Design review of the part built by this model. Coordinates are the model's own, in mm. A direction names the side the tool comes from. Coordinates: 2 decimals unless noted, no trailing zeros. Order: outer loops, then holes, each group sorted by start corner. A loop starts at its lowest first (then second) coordinate and runs counter-clockwise, first axis right, second up. Notation, with made-up numbers: (-27, 0) -> (29, 0) arc R36 cw to (29, 35) -> close; hole circle Ø1 at (69.5, -33). An arc over 180 degrees is marked (long way). Write item = value, one per line.
```python
from build123d import *

# Parameters (mm, degrees)
SKETCH1_R           = 27.5
BOSS_EXTRUDE1_DEPTH = 3
SKETCH2_R           = 27.5
SKETCH2_R_2         = 24.5
BOSS_EXTRUDE2_DEPTH = 15
SKETCH4_R           = 4
CUT_EXTRUDE1_DEPTH  = 5
SKETCH5_R           = 1.5
CUT_EXTRUDE2_DEPTH  = 10
FILLET1_R           = 2
SKETCH6_R           = 24.5
SKETCH6_R_2         = 22.5
BOSS_EXTRUDE3_DEPTH = 20


with BuildPart() as part:
    # Sketch1 → Boss-Extrude1 (new body)
    with BuildSketch(Plane(origin=(0, 0, 0), x_dir=(1, 0, 0), z_dir=(0, 1, 0))):
        with Locations(Location((0, 0, 0), (0, 0, 270))):
            Circle(SKETCH1_R)
    extrude(amount=BOSS_EXTRUDE1_DEPTH)

    # Sketch2 → Boss-Extrude2 (add)
    with BuildSketch(Plane(origin=(0, 3, 0), x_dir=(1, 0, 0), z_dir=(0, 1, 0))):
        with Locations(Location((0, 0, 0), (0, 0, 270))):
            Circle(SKETCH2_R)
        with Locations(Location((0, 0, 0), (0, 0, 270))):
            Circle(SKETCH2_R_2, mode=Mode.SUBTRACT)
    extrude(amount=BOSS_EXTRUDE2_DEPTH)

    # Sketch4 → Cut-Extrude1 (cut)
    with BuildSketch(Plane(origin=(0, 3, 0), x_dir=(1, 0, 0), z_dir=(0, 1, 0))):
        with Locations(Location((0, 0, 0), (0, 0, 270))):
            Circle(SKETCH4_R)
    extrude(amount=-CUT_EXTRUDE1_DEPTH, mode=Mode.SUBTRACT)

    # Sketch5 → Cut-Extrude2 (cut)
    with BuildSketch(Plane(origin=(0, 3, 0), x_dir=(1, 0, 0), z_dir=(0, 1, 0))):
        with BuildLine():
            Line((-2.588190451, 9.659258263), (-5.176380902, 19.318516526))
            ThreePointArc((-5.176380902, 19.318516526), (-14.142135624, 14.142135624), (-19.318516526, 5.176380902))
            Line((-19.318516526, 5.176380902), (-9.659258263, 2.588190451))
            ThreePointArc((-9.659258263, 2.588190451), (-7.071067812, 7.071067812), (-2.588190451, 9.659258263))
        make_face()
        with BuildLine():
            ThreePointArc((19.318516526, 5.176380902), (14.142135624, 14.142135624), (5.176380902, 19.318516526))
            Line((5.176380902, 19.318516526), (2.588190451, 9.659258263))
            ThreePointArc((2.588190451, 9.659258263), (7.071067812, 7.071067812), (9.659258263, 2.588190451))
            Line((9.659258263, 2.588190451), (19.318516526, 5.176380902))
        make_face()
        with BuildLine():
            Line((-9.659258263, -2.588190451), (-19.318516526, -5.176380902))
            ThreePointArc((-19.318516526, -5.176380902), (-14.142135624, -14.142135624), (-5.176380902, -19.318516526))
            Line((-5.176380902, -19.318516526), (-2.588190451, -9.659258263))
            ThreePointArc((-2.588190451, -9.659258263), (-7.071067812, -7.071067812), (-9.659258263, -2.588190451))
        make_face()
        with BuildLine():
            ThreePointArc((5.176380902, -19.318516526), (14.142135624, -14.142135624), (19.318516526, -5.176380902))
            Line((19.318516526, -5.176380902), (9.659258263, -2.588190451))
            ThreePointArc((9.659258263, -2.588190451), (7.071067812, -7.071067812), (2.588190451, -9.659258263))
            Line((2.588190451, -9.659258263), (5.176380902, -19.318516526))
        make_face()
        with Locations(Location((0, 15, 0), (0, 0, 270))):
            Circle(SKETCH5_R)
        with Locations(Location((15, 0, 0), (0, 0, 270))):
            Circle(SKETCH5_R)
        with Locations(Location((0, -15, 0), (0, 0, 270))):
            Circle(SKETCH5_R)
        with Locations(Location((-15, 0, 0), (0, 0, 270))):
            Circle(SKETCH5_R)
    extrude(amount=-CUT_EXTRUDE2_DEPTH, mode=Mode.SUBTRACT)

    # Fillet1
    fillet1_edges = [part.edges().sort_by_distance(p)[0] for p in [
        (-9.659258263, 1.5, 2.588190451),
        (-2.588190451, 1.5, 9.659258263),
        (-5.176380902, 1.5, 19.318516526),
        (-19.318516526, 1.5, 5.176380902),
        (2.588190451, 1.5, 9.659258263),
        (9.659258263, 1.5, 2.588190451),
        (19.318516526, 1.5, 5.176380902),
        (5.176380902, 1.5, 19.318516526),
        (9.659258263, 1.5, -2.588190451),
        (2.588190451, 1.5, -9.659258263),
        (5.176380902, 1.5, -19.318516526),
        (19.318516526, 1.5, -5.176380902),
        (-2.588190451, 1.5, -9.659258263),
        (-9.659258263, 1.5, -2.588190451),
        (-19.318516526, 1.5, -5.176380902),
        (-5.176380902, 1.5, -19.318516526),
    ]]
    fillet(fillet1_edges, radius=FILLET1_R)

    # Sketch6 → Boss-Extrude3 (add)
    with BuildSketch(Plane(origin=(0, 3, 0), x_dir=(1, 0, 0), z_dir=(0, 1, 0))):
        with Locations(Location((0, 0, 0), (0, 0, 270))):
            Circle(SKETCH6_R)
        with Locations(Location((0, 0, 0), (0, 0, 270))):
            Circle(SKETCH6_R_2, mode=Mode.SUBTRACT)
    extrude(amount=BOSS_EXTRUDE3_DEPTH)


solid = part.part
```
(1) We need section A-A (x = 0). Write out the cut boundary in (y, z).
Report:
outline = (0, -27.5) -> (18, -27.5) -> (18, -24.5) -> (23, -24.5) -> (23, -22.5) -> (3, -22.5) -> (3, -16.5) -> (0, -16.5) -> close; (0, -13.5) -> (3, -13.5) -> (3, -4) -> (0, -4) -> close; (0, 4) -> (3, 4) -> (3, 13.5) -> (0, 13.5) -> close; (0, 16.5) -> (3, 16.5) -> (3, 22.5) -> (23, 22.5) -> (23, 24.5) -> (18, 24.5) -> (18, 27.5) -> (0, 27.5) -> close
(2) Insertion check: pin 1 (2.5 mm diameter, centred on x = 0, z = 15, fed in from -Y); pin 2 (22.5 mm diameter, centred on x = 1.5, z = -2, fed in from +Y); pin 3 (3 mm diameter, centred on y = 7.5, z = -8, fed in from +X); pin 4 (1.5 mm diameter, centred on y = 4.5, z = -15.5, fed in from -X). Each pin has a flat end and moves straight along its axis. Give the tip position at first contact, or say it passes through.
Report:
pin_1 = through
pin_2 = 3
pin_3 = 26.72
pin_4 = -23.21
(3) We need section B-B (z = 0). Write out the cut boundary in (x, y), and give its area (3 significant figures).
Report:
outline = (-27.5, 0) -> (-16.5, 0) -> (-16.5, 3) -> (-22.5, 3) -> (-22.5, 23) -> (-24.5, 23) -> (-24.5, 18) -> (-27.5, 18) -> close; (-13.5, 0) -> (-4, 0) -> (-4, 3) -> (-13.5, 3) -> close; (4, 0) -> (13.5, 0) -> (13.5, 3) -> (4, 3) -> close; (16.5, 0) -> (27.5, 0) -> (27.5, 18) -> (24.5, 18) -> (24.5, 23) -> (22.5, 23) -> (22.5, 3) -> (16.5, 3) -> close
area = 293 mm²
(4) The part is to be moulded in two halves that separate along X. For faces 3 (the flat face through (-2, 18, -25)), 4 (the flat face through (3.835, 1.521, 14.313)), 5 (the flat face through (-3.835, 1.521, -14.313)), say which applies: released by +X, released by -X, zero draft, split by the parting line, or undercut.
Report:
face_3 = zero draft
face_4 = undercut
face_5 = undercut
(5) For faces 1 (the cylindrical face through (-5.639, 1.479, -18.536)), 2 (the flat face through (0, 3, 5)), list the 3-axis set-ups (+Z, -Z, +X, -X, +Y, -Y) from which the entire face can be reached by the end or side of a thin tool; tool diameter is ignored.
Report:
face_1 = +Y, -Y
face_2 = +Y
(6) We need section C-C (y = 9). Write out the cut boundary in (x, z).
Report:
outline = circle Ø55 at (0, 0); hole circle Ø45 at (0, 0)
(7) We need section D-D (z = 10.5). Write out the cut boundary in (x, y).
Report:
outline = (-25.42, 0) -> (-17.02, 0) -> (-17.02, 3) -> (-19.9, 3) -> (-19.9, 23) -> (-22.14, 23) -> (-22.14, 18) -> (-25.42, 18) -> close; (-3.04, 0) -> (3.04, 0) -> (3.04, 3) -> (-3.04, 3) -> close; (17.02, 0) -> (25.42, 0) -> (25.42, 18) -> (22.14, 18) -> (22.14, 23) -> (19.9, 23) -> (19.9, 3) -> (17.02, 3) -> close
(8) For L1, parallel to X at y = 1.5, z = 0; L2, parallel to X at y = 0.8, z = -15; L3, parallel to X at y = 15, z = 0, list the stretches that pass through material, from the lowest coordinate up.
Report:
L1 = -27.5 to -16.5, -13.5 to -4, 4 to 13.5, 16.5 to 27.5
L2 = -23.05 to -13.23, -4.02 to -1.5, 1.5 to 4.02, 13.23 to 23.05
L3 = -27.5 to -22.5, 22.5 to 27.5
